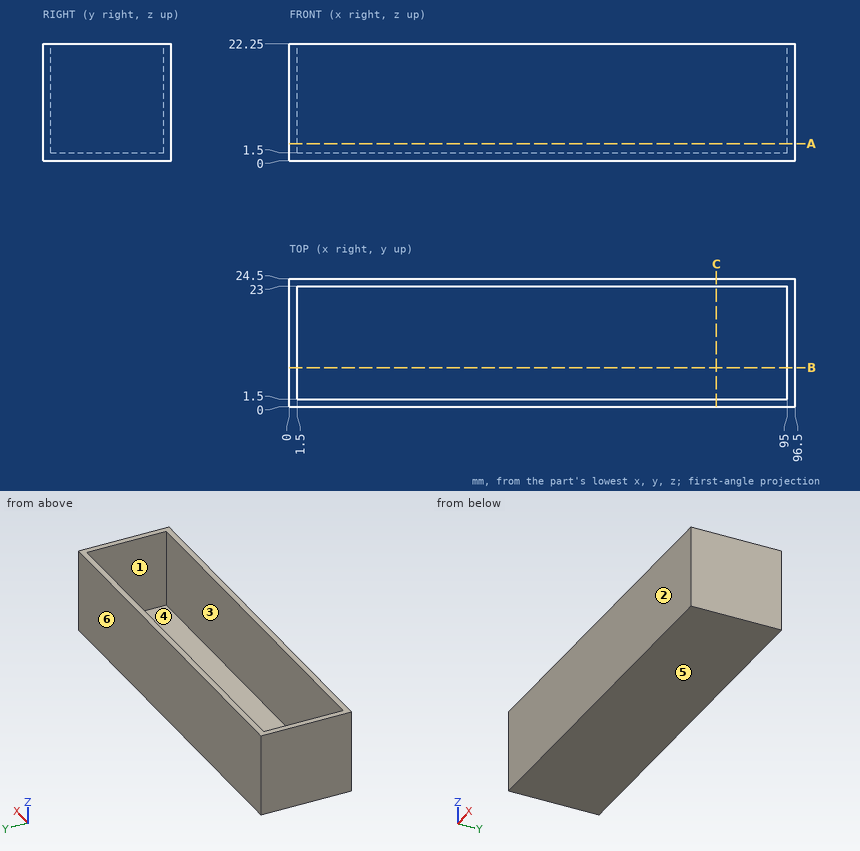
Design review of the part shown in the three views and the two pictorial views. Dimensions are in mm from the part's minimum x, y and z. A direction names the side the tool comes from. Coordinates: 2 decimals unless noted, no trailing zeros. Order: outer loops, then holes, each group sorted by start corner. A loop starts at its lowest first (then second) coordinate and runs counter-clockwise, first axis right, second up.
1) Wall thickness on line 1 along Y through (x, z) = (38.5, 21.25); line 2 along X through (y, z) = (12.25, 12); line 3 along Z through (x, y) = (69.5, 10): over which ranges is each line inside the solid? List them lowest first.
2) For the marked faces 1 and 2, list the 3-axis set-ups (+Z, -Z, +X, -X, +Y, -Y) from which the entire face can be reached by the end or side of a thin tool; tool diameter is ignored.
3) Take a section at B-B, the plane y = 7.5. Give the boundary of the cut face in (x, z), and give its area (3 significant figures).
4) Clearance check with flat-ended pins moving along their axes: pin 1 (10 mm diameter, centred on x = 44.5, y = 3, fed in from +Z); pin 2 (6 mm diameter, centred on x = 35.5, y = 7.5, fed in from +Z). State where each tip first meets the part, or that it passes through.
5) Take a section at C-C, the plane x = 81.5. Give the boundary of the cut face in (y, z), and give its area (3 significant figures).
6) Take a section at A-A, the plane z = 3.25. Give the boundary of the cut face in (x, y), and give its area (3 significant figures).
7) Mouldability with a two-part tool opening along Y and no side actions: class the marked faces 3, 4, 5 and 6 as +Y half, -Y half, draft (parallel to the pull), parting line (faces both ways), or undercut.
Returned:
1. line 1: y = 0 to 1.5, 23 to 24.5
1. line 2: x = 0 to 1.5, 95 to 96.5
1. line 3: z = 0 to 1.5
2. face 1: +Z
2. face 2: +Z, -Z, +X, -X, -Y
3. outline: (0, 0) - (96.5, 0) - (96.5, 22.25) - (95, 22.25) - (95, 1.5) - (1.5, 1.5) - (1.5, 22.25) - (0, 22.25) - close
3. area: 207 mm2
4. pin 1: stops at z = 22.25
4. pin 2: stops at z = 1.5
5. outline: (0, 0) - (24.5, 0) - (24.5, 22.25) - (23, 22.25) - (23, 1.5) - (1.5, 1.5) - (1.5, 22.25) - (0, 22.25) - close
5. area: 99.0 mm2
6. outline: (0, 0) - (96.5, 0) - (96.5, 24.5) - (0, 24.5) - close; hole (1.5, 1.5) - (95, 1.5) - (95, 23) - (1.5, 23) - close
6. area: 354 mm2
7. face 3: undercut
7. face 4: undercut
7. face 5: draft
7. face 6: +Y half
